Can you work these out from the model? Positions are in its coordinate system, mm. Face numbers are marked on the shaded views. A direction names the side the tool comes from. Give positions to 0.01 mm unless a question says otherwise; leave off trailing zeros. Order: outer loops, then holes, each group sorted by start corner. A loop starts at its lowest first (then second) coordinate and runs counter-clockwise, first axis right, second up. Notation, with made-up numbers: M 71.25,-24 L 101.25,-24 A17 ccw 101.25,7 Z; hole C 7.25,15.5 d6. An arc over 180 degrees is marked long. One line per question, with ' | ' between items. Start each with the question number.
1) If we section it at A-A, the plane z = 0: Please give me the cut outline in (x, y), plus the area to 3 significant figures.
2) For the marked faces 1 and 2, which set-ups out of +Z, -Z, +X, -X, +Y, -Y let a thin tool reach every point of the face, with its end or its side?
3) If we section it at C-C, the plane x = 4.75: Please give me the cut outline in (y, z).
4) If we section it at D-D, the plane z = 6: Please give me the cut outline in (x, y), plus the area to 3 significant figures.
5) If we section it at B-B, the plane y = -38.5: Please give me the cut outline in (x, z), plus the area to 3 significant figures.
6) Please list where these lines run through material, in increasing order: line 1 along Y through (x, z) = (5.25, -1.5); line 2 along X through (y, z) = (-1.5, -1.25); line 3 along Y through (x, z) = (1.75, -3.5). Write a range as [from, to].
7) I'm going to push flat-ended pins straight in: pin 1 Ø3 at (y, z) = (-29, -2) entering from -X; pin 2 Ø5 at (x, z) = (3, 2) entering from -Y. Where does each tip first touch, or does it pass through?
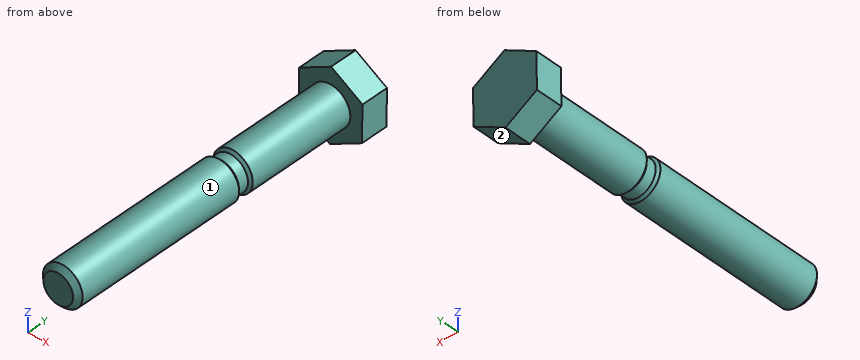
```python
from build123d import *

# Parameters (mm, degrees)
BOSS_EXTRUDE1_DEPTH = 5.4
SKETCH3_R           = 4
BOSS_EXTRUDE2_DEPTH = 60
SKETCH4_R           = 4.399457614
SKETCH4_R_2         = 3.503217006
CUT_EXTRUDE1_DEPTH  = 1
CHAMFER1_SIZE       = 0.5
CHAMFER2_SIZE       = 1


with BuildPart() as part:
    # Sketch1 → Boss-Extrude1 (new body)
    with BuildSketch(Plane(origin=(0, 0, 0), x_dir=(1, 0, 0), z_dir=(0, 1, 0))):
        Polygon((6.457637206, -3.593362639), (6.340761933, 3.795796549), (-0.116875273, 7.389159188), (-6.457637206, 3.593362639), (-6.340761933, -3.795796549), (0.116875273, -7.389159188), align=None)
    extrude(amount=BOSS_EXTRUDE1_DEPTH)

    # Sketch3 → Boss-Extrude2 (add)
    with BuildSketch(Plane.XZ):
        with Locations(Location((0, 0, 0), (0, 0, 90))):
            Circle(SKETCH3_R)
    extrude(amount=BOSS_EXTRUDE2_DEPTH)

    # Sketch4 → Cut-Extrude1 (cut, symmetric)
    with BuildSketch(Plane(origin=(0, -23, 0), x_dir=(-1, 0, 0), z_dir=(0, -1, 0))):
        Circle(SKETCH4_R)
        with Locations(Location((0, 0, 0), (0, 0, 90))):
            Circle(SKETCH4_R_2, mode=Mode.SUBTRACT)
    extrude(amount=CUT_EXTRUDE1_DEPTH, both=True, mode=Mode.SUBTRACT)

    # Chamfer1
    # the kernel refuses this chamfer: 0.5 mm, written as the material it takes off along each edge
    with BuildSketch(Plane(origin=(0, -22, 0), x_dir=(0, 0, 1), z_dir=(-1, 0, 0))) as chamfer1_piece_1_section:
        Polygon((4, CHAMFER1_SIZE), (4 - CHAMFER1_SIZE, 0), (4, 0), align=None)
    chamfer1_piece_1 = revolve(axis=Axis((0, -22, 0), (0, 1, 0)), mode=Mode.PRIVATE)
    chamfer1_piece_1 = chamfer1_piece_1 - Plane(origin=(0, -21.751856144, 0), x_dir=(0, 0, -1), z_dir=(0, 1, 0)) * Cylinder(3.503217006, 16, mode=Mode.PRIVATE)
    add(chamfer1_piece_1, mode=Mode.SUBTRACT)
    with BuildSketch(Plane(origin=(0, -24, 0), x_dir=(0, 0, 1), z_dir=(-1, 0, 0))) as chamfer1_piece_2_section:
        Polygon((4 - CHAMFER1_SIZE, 0), (4, -CHAMFER1_SIZE), (4, 0), align=None)
    chamfer1_piece_2 = revolve(axis=Axis((0, -24, 0), (0, 1, 0)), mode=Mode.PRIVATE)
    chamfer1_piece_2 = chamfer1_piece_2 - Plane(origin=(0, -24.248143856, 0), x_dir=(0, 0, -1), z_dir=(0, 1, 0)) * Cylinder(3.503217006, 16, mode=Mode.PRIVATE)
    add(chamfer1_piece_2, mode=Mode.SUBTRACT)

    # Chamfer2
    chamfer2_edges = [part.edges().sort_by_distance(p)[0] for p in [
        (0, -60, -4),
    ]]
    chamfer(chamfer2_edges, length=CHAMFER2_SIZE)


solid = part.part
```
Results found:
1) outline: M -6.4,0 L -4,0 L -4,-21.5 L -3.5,-22 L -3.5,-24 L -4,-24.5 L -4,-59 L -3,-60 L 3,-60 L 4,-59 L 4,-24.5 L 3.5,-24 L 3.5,-22 L 4,-21.5 L 4,0 L 6.4,0 L 6.4,5.4 L -6.4,5.4 Z | area: 546 mm²
2) face 1: -Y | face 2: -Z, +X, +Y, -Y
3) outline: M 0,-4.68 L 5.4,-4.68 L 5.4,4.62 L 0,4.62 Z
4) outline: M -2.38,0 L 2.44,0 L 2.44,5.4 L -2.38,5.4 Z | area: 26.0 mm²
5) outline: C 0,0 d8 | area: 50.3 mm²
6) line 1: y = [0, 5.4] | line 2: x = [-3.8, 3.8] | line 3: y = [-59.09, -24.41], [-21.59, 5.4]
7) pin 1: stops at x = -3.97 | pin 2: stops at y = -60
